```python
from build123d import *

# Parameters (mm, degrees)
CROQUIS1_W              = 37.5
CROQUIS1_H              = 36
SALIENTE_EXTRUIR1_DEPTH = 1.8
CROQUIS2_W              = 27.5
CROQUIS2_H              = 26
SALIENTE_EXTRUIR2_DEPTH = 3
CROQUIS3_W              = 21
CROQUIS3_H              = 2.54
SALIENTE_EXTRUIR3_DEPTH = 2.6
CROQUIS4_W              = 0.8
CROQUIS4_H              = 0.8
SALIENTE_EXTRUIR4_DEPTH = 6
CROQUIS5_R              = 4
SALIENTE_EXTRUIR5_DEPTH = 40


with BuildPart() as part:
    # Croquis1 → Saliente-Extruir1 (new body)
    with BuildSketch(Plane(origin=(0, 0, 0), x_dir=(1, 0, 0), z_dir=(0, 1, 0))):
        with Locations((18.75, 18)):
            Rectangle(CROQUIS1_W, CROQUIS1_H)
    extrude(amount=SALIENTE_EXTRUIR1_DEPTH)

    # Croquis2 → Saliente-Extruir2 (add)
    with BuildSketch(Plane(origin=(0, 1.8, 0), x_dir=(1, 0, 0), z_dir=(0, 1, 0))):
        with Locations((18.75, 18)):
            Rectangle(CROQUIS2_W, CROQUIS2_H)
    extrude(amount=SALIENTE_EXTRUIR2_DEPTH)

    # Croquis3 → Saliente-Extruir3 (add)
    with BuildSketch(Plane(origin=(37.5, 0, 0), x_dir=(0, 0, -1), z_dir=(1, 0, 0))):
        with Locations((18, -0.27)):
            Rectangle(CROQUIS3_W, CROQUIS3_H)
    extrude(amount=SALIENTE_EXTRUIR3_DEPTH)

    # Croquis4 → Saliente-Extruir4 (add)
    with BuildSketch(Plane(origin=(40.1, 0, 0), x_dir=(0, 0, -1), z_dir=(1, 0, 0))):
        with Locations((21.81, -0.27)):
            Rectangle(CROQUIS4_W, CROQUIS4_H)
        with Locations((19.27, -0.27)):
            Rectangle(CROQUIS4_W, CROQUIS4_H)
        with Locations((16.73, -0.27)):
            Rectangle(CROQUIS4_W, CROQUIS4_H)
        with Locations((24.35, -0.27)):
            Rectangle(CROQUIS4_W, CROQUIS4_H)
        with Locations((26.89, -0.27)):
            Rectangle(CROQUIS4_W, CROQUIS4_H)
        with Locations((14.19, -0.27)):
            Rectangle(CROQUIS4_W, CROQUIS4_H)
        with Locations((11.65, -0.27)):
            Rectangle(CROQUIS4_W, CROQUIS4_H)
        with Locations((9.11, -0.27)):
            Rectangle(CROQUIS4_W, CROQUIS4_H)
    extrude(amount=SALIENTE_EXTRUIR4_DEPTH)

    # Croquis5 → Saliente-Extruir5 (add)
    with BuildSketch(Plane.ZY):
        with Locations((-10, 1.8)):
            Circle(CROQUIS5_R)
    extrude(amount=SALIENTE_EXTRUIR5_DEPTH)


solid = part.part
```
Part model, mm, in its own coordinate system. A direction names the side the tool comes from. Give positions to 0.01 mm unless a question says otherwise; leave off trailing zeros. Order: outer loops, then holes, each group sorted by start corner. A loop starts at its lowest first (then second) coordinate and runs counter-clockwise, first axis right, second up. Notation, with made-up numbers: M 0,77 L 45,77 A36 cw 45,116 Z; hole C 30.5,-31 d2. An arc over 180 degrees is marked long. Use a Markdown table: item, result. Add a question column.
(1) Saw through at B-B, the plane x = 18. Give the cut face in (y, z), and give its area (3 significant figures).
(2) 3-axis set-ups, long thin cutter, end or side, ignore diameter. For faces 5 (the face through (39, 1, -18)), 6 (the face through (19, 3, -5)), 7 (the face through (0, 3, -10)), 8 (the face through (0, -1, -10)): which of +Z, -Z, +X, -X, +Y, -Y reach the whole face in a straight line?
(3) Saw through at A-A, the plane y = 3.25. Give the cut face in (x, z).
(4) Saw through at D-D, the plane x = 38.5. Give the cut face in (y, z), and give its area (3 significant figures).
(5) Drop flat-ended pins along their axis: P1, Ø2, axis at y = 1, z = -3, coming from the -X side; P2, Ø3, axis at x = 23.5, z = -4.5, coming from the +Y side; P3, Ø0.6, axis at x = 42, z = -16.5, coming from the -Y side. Give the stop position or say it passes through.
(6) Mould opens along Z. For faces 1 (the face through (32.5, 3, -18)), 2 (the face through (40.1, 0, -18)), 3 (the face through (-19.7, -0.6, -13.2)), 4 (the face through (19, 3, -31)) say: +Z half, -Z half, draft (parallel to the pull), parting line (faces both ways), or undercut.
(7) Probe line 1 along X through (y, z) = (2.5, -8); line 2 along Y through (x, z) = (24.5, -7); line 3 along X through (y, z) = (2.25, -21). List the from-to ranges inside material, lowest first. Write a range as [from, to].
(8) Saw through at C-C, the plane z = -2. Give the cut face in (x, y).
Answer key:
| question | item | result |
|---|---|---|
| 1 | outline | M 0,-36 L 1.8,-36 L 1.8,-31 L 4.8,-31 L 4.8,-5 L 1.8,-5 L 1.8,0 L 0,0 Z |
| 1 | area | 143 mm^2 |
| 2 | face 5 | +Z, -Z, +X, +Y |
| 2 | face 6 | +Z, +X, -X, +Y |
| 2 | face 7 | +Z, -Z, +Y |
| 2 | face 8 | +Z, -Z, -Y |
| 3 | outline | M -40,-13.73 L 0,-13.73 L 0,-6.27 L -40,-6.27 Z; M 5,-31 L 32.5,-31 L 32.5,-5 L 5,-5 Z |
| 4 | outline | M -1.54,-28.5 L 1,-28.5 L 1,-7.5 L -1.54,-7.5 Z |
| 4 | area | 53.3 mm^2 |
| 5 | P1 | x = 0 |
| 5 | P2 | y = 4.8 |
| 5 | P3 | y = -0.67 |
| 6 | face 1 | draft |
| 6 | face 2 | undercut |
| 6 | face 3 | parting line |
| 6 | face 4 | -Z half |
| 7 | line 1 | [-40, 0], [5, 32.5] |
| 7 | line 2 | [0, 4.8] |
| 7 | line 3 | [5, 32.5] |
| 8 | outline | M 0,0 L 37.5,0 L 37.5,1.8 L 0,1.8 Z |
